Build history of the part. All positions in model axes, mm. A direction names the side the tool comes from. Coordinates: 2 decimals unless noted, no trailing zeros. Order: outer loops, then holes, each group sorted by start corner. A loop starts at its lowest first (then second) coordinate and runs counter-clockwise, first axis right, second up. Notation, with made-up numbers: (15, -9.75) - (30, -9.75) arc R16 cw to (30, -5.75) - close; hole circle Ø2 at (11.5, 42). An arc over 180 degrees is marked (long way). One line per item, written item: value.
from build123d import *

# Parameters (mm, degrees)
F0_W     = 60
F0_H     = 20
F1_DEPTH = 3
F2_W     = 4
F2_H     = 20
F3_DEPTH = 25
F4_W     = 60
F4_H     = 25
F5_DEPTH = 5


# Not quite as in the source:
# - a pattern or mirror of a feature is missing from the dataset's text; its kind, count and spacing are read off the source's solid


with BuildPart() as f1:
    # F0 (on Top) → F1 (new body)
    with BuildSketch(Plane.XY):
        Rectangle(F0_W, F0_H)
    extrude(amount=F1_DEPTH)

    # F2 (on face) → F3 (join)
    with BuildSketch(Plane.XY.offset(3)):
        with Locations((-28, 0)):
            Rectangle(F2_W, F2_H)
    f3 = extrude(amount=F3_DEPTH)

    # F3_copies: F3 across plane
    add(f3.mirror(Plane(origin=(0, 0, 0), x_dir=(0, 0, 1), z_dir=(1, 0, 0))))

    # F4 (on Front) → F5 (cut, symmetric)
    with BuildSketch(Plane.XZ):
        with Locations((0, 15.5)):
            Rectangle(F4_W, F4_H)
    extrude(amount=F5_DEPTH, both=True, mode=Mode.SUBTRACT)


solid = f1.part
1. Two-plate mould, pull along X, no slides. Class faces 1 (the face through (-26, 7, 15)), 2 (the face through (0, 0, 0)), 3 (the face through (30, -7, 14)): pulls with the +X half, pulls with the -X half, needs draft (parallel to the pull), parting line crosses it, or undercut.
Values found:
face 1: undercut
face 2: needs draft
face 3: pulls with the +X half
2. Band-saw the part on A-A, the plane z = 20.5. Give the cut face in (x, y).
Values found:
outline: (-30, -10) - (-26, -10) - (-26, -5) - (-30, -5) - close; (-30, 5) - (-26, 5) - (-26, 10) - (-30, 10) - close; (26, -10) - (30, -10) - (30, -5) - (26, -5) - close; (26, 5) - (30, 5) - (30, 10) - (26, 10) - close
3. Band-saw the part on C-C, the plane x = 3. Give the cut face in (y, z), and give its area (3 significant figures).
Values found:
outline: (-10, 0) - (10, 0) - (10, 3) - (-10, 3) - close
area: 60.0 mm2
4. Flat gauge pins, fed straight in: P1, Ø8, axis at x = 0, y = -4, coming from the +Z side; P2, Ø1.5, axis at y = -1.5, z = 4.5, coming from the +X side. Where does each tip first touch, or does it go through?
Values found:
P1: stops at z = 3
P2: passes through
5. Band-saw the part on D-D, the plane y = -2.75. Give the cut face in (x, z), and give its area (3 significant figures).
Values found:
outline: (-30, 0) - (30, 0) - (30, 3) - (-30, 3) - close
area: 180 mm2
6. Band-saw the part on B-B, the plane y = -6.75. Give the cut face in (x, z).
Values found:
outline: (-30, 0) - (30, 0) - (30, 28) - (26, 28) - (26, 3) - (-26, 3) - (-26, 28) - (-30, 28) - close
7. 3-axis set-ups, long thin cutter, end or side, ignore diameter. For faces 4 (the face through (-28, -5, 16)), 5 (the face through (-28, 8, 28)), 6 (the face through (26, -8, 15)): which of +Z, -Z, +X, -X, +Y, -Y reach the whole face in a straight line?
Values found:
face 4: +Z, +X, -X
face 5: +Z, +X, -X, +Y, -Y
face 6: +Z, +Y, -Y
8. Probe line 1 along Y through (x, z) = (27.5, 19); line 2 along X through (y, z) = (6.5, 20.5); line 3 along Z through (x, y) = (-14, 5). List the from-to ranges inside material, lowest first.
Values found:
line 1: y = -10 to -5, 5 to 10
line 2: x = -30 to -26, 26 to 30
line 3: z = 0 to 3
